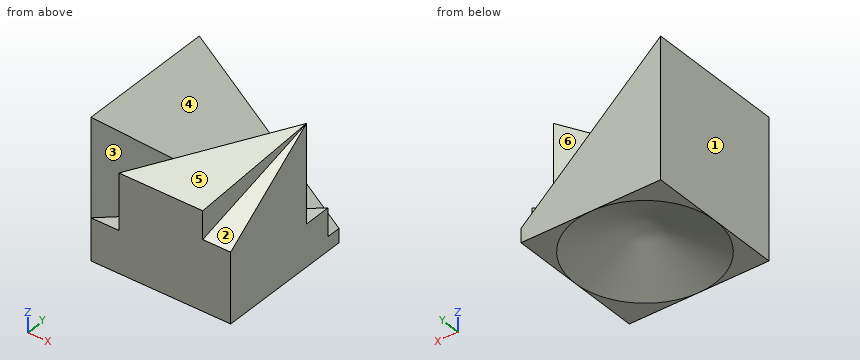
```python
from build123d import *

# Parameters (mm, degrees)
F0_W      = 50
F0_H      = 50
F1_DEPTH  = 50
F4_DEPTH  = 35
F10_REACH = 117.2691203354


with BuildPart() as f1:
    # F0 (on Top) → F1 (new body)
    with BuildSketch(Plane.XY):
        Rectangle(F0_W, F0_H)
    extrude(amount=F1_DEPTH)

    # F3 (on face) → F4 (cut, through all)
    with BuildSketch(Plane.XY.offset(50)):
        Polygon((25, 20), (-25, -25), (-15, -25), (25, 10), align=None)
    extrude(amount=-F4_DEPTH, mode=Mode.SUBTRACT)

    # F5 (on Front) → F6 (revolve, cut)
    with BuildSketch(Plane.XZ):
        Polygon((0, 10), (0, 0), (25, 0), align=None)
    revolve(axis=Axis((0, 0, 5), (0, 0, 1)), mode=Mode.SUBTRACT)

    # F7 (on face) → F8 section 0
    with BuildSketch(Plane.XZ.offset(25), mode=Mode.PRIVATE) as f8_s0:
        Polygon((25, 50), (-15, 50), (-15, 35), (15, 35), (15, 25), (25, 25), align=None)
    loft([f8_s0.sketch, Vertex(25, 10, 50)], mode=Mode.SUBTRACT)

    f10_end = Plane(origin=(0, -2.5, 32.5), x_dir=(-0.7432941462, -0.6689647316, 0), z_dir=(0.6689647316, -0.7432941462, 0))
    # F9 (on face) → F10 (cut, up to a plane its end follows)
    with BuildSketch(Plane(origin=(0, 25, 0), x_dir=(-1, 0, 0), z_dir=(0, 1, 0))):
        Polygon((-25, 5), (25, 50), (-25, 50), align=None)
    f10_long = extrude(amount=-F10_REACH, mode=Mode.PRIVATE)
    add(split(f10_long, bisect_by=f10_end, keep=Keep.BOTTOM, mode=Mode.PRIVATE), mode=Mode.SUBTRACT)


solid = f1.part
```
Verification items for the finished model (mm, model axes). Face numbers are marked on the shaded views. A direction names the side the tool comes from. Round coordinates to 2 decimals unless told otherwise and drop trailing zeros. Write each loop counter-clockwise with the first axis right and the second up, starting at its lowest first coordinate (ties: lowest second). Pieces come first, ordered by that corner, then holes.
1. Section check A-A on z = 11. Enter the section's corners in (x, y).
2. Draft check along Y on the marked faces 4, 5 and 6. Enter one of: +Y half, -Y half, draft (parallel to the pull), parting line (faces both ways), or undercut.
3. Access from +Z, -Z, +X, -X, +Y, -Y to the whole of each face (thin tool, end or side, straight path). Record for the marked faces 1, 2 and 3.
4. Gauge pin test, flat ends, axial feed: P1, Ø6, axis at x = -14.5, y = -13, coming from the +Z side; P2, Ø6, axis at x = -16.5, y = 18, coming from the +Z side; P3, Ø2, axis at y = 17.5, z = 32.5, coming from the +X side. Record the tip position at first contact, or that the pin passes through.
5. Scan lines: L1, parallel to X at y = 16.5, z = 11; L2, parallel to X at y = 7.5, z = 34; L3, parallel to X at y = 21.5, z = 14. Record each from-to range of solid material in increasing order.
Answer:
1. outline: (-25, -25) - (25, -25) - (25, 20) - (18.33, 14) - (18.33, 25) - (-25, 25) - close
2. face 4: draft
2. face 5: -Y half
2. face 6: undercut
3. face 1: +Z, -Z, -X, +Y, -Y
3. face 2: +Z, +X, -Y
3. face 3: +Z
4. P1: stops at z = 43.25
4. P2: stops at z = 45.05
4. P3: stops at x = -4.44
5. L1: x = -25 to 18.33, 21.11 to 25
5. L2: x = -25 to -7.22, 22.14 to 25
5. L3: x = -25 to 15
